Here's how the part is built. I have some questions about the finished solid (model axes, mm). A direction names the side the tool comes from. Give positions to 0.01 mm unless a question says otherwise; leave off trailing zeros. Loops run counter-clockwise (first coordinate to the right, second up) from the corner with the lowest first, then second, coordinate; pieces in that order, holes last. Notation, with made-up numbers: (-37, 68.5) - (0, 68.5) arc R27 ccw to (0, 87.5) - close; hole circle Ø9 at (84.5, 36). An arc over 180 degrees is marked (long way). Use one line per item in the form item = value.
from build123d import *

# Parameters (mm, degrees)
BOSS_EXTRUDE1_DEPTH = 72.4
BOSS_EXTRUDE2_DEPTH = 7.3
BOSS_EXTRUDE3_DEPTH = 4.3
SKETCH4_R           = 25
BOSS_EXTRUDE4_DEPTH = 6.5
SKETCH5_R           = 3.25
CUT_EXTRUDE1_DEPTH  = 3
CUT_EXTRUDE2_DEPTH  = 1
SKETCH7_R           = 1.5
CUT_EXTRUDE3_DEPTH  = 1
SKETCH8_R           = 20
CUT_EXTRUDE4_DEPTH  = 10


with BuildPart() as part:
    # Sketch1 → Boss-Extrude1 (new body)
    with BuildSketch(Plane(origin=(0, 0, 0), x_dir=(1, 0, 0), z_dir=(0, 1, 0))):
        with BuildLine():
            ThreePointArc((69.840771002, 70.864970002), (39.3, 72.2), (8.759228998, 70.864970002))
            ThreePointArc((8.759228998, 70.864970002), (3.821292476, 68.573105669), (1.493169033, 63.652160592))
            ThreePointArc((1.493169033, 63.652160592), (0.466996736, 49.89123235), (0, 36.1))
            ThreePointArc((0, 36.1), (0.466996736, 22.30876765), (1.493169033, 8.547839408))
            ThreePointArc((1.493169033, 8.547839408), (3.821292476, 3.626894331), (8.759228998, 1.335029998))
            ThreePointArc((8.759228998, 1.335029998), (39.3, 0), (69.840771002, 1.335029998))
            ThreePointArc((69.840771002, 1.335029998), (74.778707524, 3.626894331), (77.106830967, 8.547839408))
            ThreePointArc((77.106830967, 8.547839408), (78.133003264, 22.30876765), (78.6, 36.1))
            ThreePointArc((78.6, 36.1), (78.133003264, 49.89123235), (77.106830967, 63.652160592))
            ThreePointArc((77.106830967, 63.652160592), (74.778707524, 68.573105669), (69.840771002, 70.864970002))
        make_face()
    extrude(amount=BOSS_EXTRUDE1_DEPTH)

    # Sketch2 → Boss-Extrude2 (add)
    with BuildSketch(Plane(origin=(0, 72.4, 0), x_dir=(1, 0, 0), z_dir=(0, 1, 0))):
        with BuildLine():
            ThreePointArc((69.66625231, 68.872598745), (39.3, 70.2), (8.93374769, 68.872598745))
            ThreePointArc((8.93374769, 68.872598745), (5.230295298, 67.153700495), (3.484202716, 63.462991687))
            ThreePointArc((3.484202716, 63.462991687), (2.464800099, 49.796540149), (2.000184882, 36.1))
            ThreePointArc((2.000184882, 36.1), (2.464800099, 22.403459851), (3.484202716, 8.737008313))
            ThreePointArc((3.484202716, 8.737008313), (5.230295298, 5.046299505), (8.93374769, 3.327401255))
            ThreePointArc((8.93374769, 3.327401255), (39.3, 2), (69.66625231, 3.327401255))
            ThreePointArc((69.66625231, 3.327401255), (73.369704702, 5.046299505), (75.115797284, 8.737008313))
            ThreePointArc((75.115797284, 8.737008313), (76.135199901, 22.403459851), (76.599815118, 36.1))
            ThreePointArc((76.599815118, 36.1), (76.135199901, 49.796540149), (75.115797284, 63.462991687))
            ThreePointArc((75.115797284, 63.462991687), (73.369704702, 67.153700495), (69.66625231, 68.872598745))
        make_face()
    extrude(amount=BOSS_EXTRUDE2_DEPTH)

    # Sketch3 → Boss-Extrude3 (add)
    with BuildSketch(Plane.XZ):
        with BuildLine():
            ThreePointArc((69.66625231, -3.327401255), (39.3, -2), (8.93374769, -3.327401255))
            ThreePointArc((8.93374769, -3.327401255), (5.230295298, -5.046299505), (3.484202716, -8.737008313))
            ThreePointArc((3.484202716, -8.737008313), (2.464800099, -22.403459851), (2.000184882, -36.1))
            ThreePointArc((2.000184882, -36.1), (2.464800099, -49.796540149), (3.484202716, -63.462991687))
            ThreePointArc((3.484202716, -63.462991687), (5.230295298, -67.153700495), (8.93374769, -68.872598745))
            ThreePointArc((8.93374769, -68.872598745), (39.3, -70.2), (69.66625231, -68.872598745))
            ThreePointArc((69.66625231, -68.872598745), (73.369704702, -67.153700495), (75.115797284, -63.462991687))
            ThreePointArc((75.115797284, -63.462991687), (76.135199901, -49.796540149), (76.599815118, -36.1))
            ThreePointArc((76.599815118, -36.1), (76.135199901, -22.403459851), (75.115797284, -8.737008313))
            ThreePointArc((75.115797284, -8.737008313), (73.369704702, -5.046299505), (69.66625231, -3.327401255))
        make_face()
    extrude(amount=BOSS_EXTRUDE3_DEPTH)

    # Sketch4 → Boss-Extrude4 (add)
    with BuildSketch(Plane.XZ.offset(4.3)):
        with Locations((39.3, -36.1)):
            Circle(SKETCH4_R)
    extrude(amount=BOSS_EXTRUDE4_DEPTH)

    # Sketch5 → Cut-Extrude1 (cut)
    with BuildSketch(Plane(origin=(0, 79.7, 0), x_dir=(1, 0, 0), z_dir=(0, 1, 0))):
        with Locations((69.3, 58.6)):
            Circle(SKETCH5_R)
        with Locations((69.3, 13.6)):
            Circle(SKETCH5_R)
        with Locations((9.3, 13.6)):
            Circle(SKETCH5_R)
        with Locations((9.3, 58.6)):
            Circle(SKETCH5_R)
    extrude(amount=-CUT_EXTRUDE1_DEPTH, mode=Mode.SUBTRACT)

    # Sketch6 → Cut-Extrude2 (cut)
    with BuildSketch(Plane(origin=(0, 79.7, 0), x_dir=(1, 0, 0), z_dir=(0, 1, 0))):
        with BuildLine():
            Line((10.8, 54.1), (67.8, 54.1))
            ThreePointArc((67.8, 54.1), (69.567766953, 53.367766953), (70.3, 51.6))
            Line((70.3, 51.6), (70.3, 20.6))
            ThreePointArc((70.3, 20.6), (69.567766953, 18.832233047), (67.8, 18.1))
            Line((67.8, 18.1), (10.8, 18.1))
            ThreePointArc((10.8, 18.1), (9.032233047, 18.832233047), (8.3, 20.6))
            Line((8.3, 20.6), (8.3, 51.6))
            ThreePointArc((8.3, 51.6), (9.032233047, 53.367766953), (10.8, 54.1))
        make_face()
    extrude(amount=-CUT_EXTRUDE2_DEPTH, mode=Mode.SUBTRACT)

    # Sketch7 → Cut-Extrude3 (cut)
    with BuildSketch(Plane(origin=(0, 79.7, 0), x_dir=(1, 0, 0), z_dir=(0, 1, 0))):
        with Locations((32.8, 12.1)):
            Circle(SKETCH7_R)
        with Locations((45.8, 12.1)):
            Circle(SKETCH7_R)
    extrude(amount=-CUT_EXTRUDE3_DEPTH, mode=Mode.SUBTRACT)

    # Sketch8 → Cut-Extrude4 (cut)
    with BuildSketch(Plane.XZ.offset(10.8)):
        with Locations((39.3, -36.1)):
            Circle(SKETCH8_R)
    extrude(amount=-CUT_EXTRUDE4_DEPTH, mode=Mode.SUBTRACT)


solid = part.part
(1) For P1, Ø2.5, axis at x = 32.8, z = -12.1, coming from the +Y side; P2, Ø0.8, axis at x = 48.5, y = 79, coming from the -Z side; P3, Ø12, axis at x = 40.5, z = -35.5, coming from the -Y side, each with a flat end and sliding along its axis, tell me the tip position at first contact or that it passes through.
Geometry says:
P1 = 78.7
P2 = -70.09
P3 = -0.8
(2) If we section it at A-A (x = 39.3): List the corners of the cut face in (y, z) for me.
Geometry says:
outline = (-10.8, -61.1) - (-4.3, -61.1) - (-4.3, -70.2) - (0, -70.2) - (0, -72.2) - (72.4, -72.2) - (72.4, -70.2) - (79.7, -70.2) - (79.7, -54.1) - (78.7, -54.1) - (78.7, -18.1) - (79.7, -18.1) - (79.7, -2) - (72.4, -2) - (72.4, 0) - (0, 0) - (0, -2) - (-4.3, -2) - (-4.3, -11.1) - (-10.8, -11.1) - (-10.8, -16.1) - (-0.8, -16.1) - (-0.8, -56.1) - (-10.8, -56.1) - close
(3) For faces 5 (the cylindrical face through (36.045, -7.504, -11.313)), 6 (the cylindrical face through (72.4, 78.22, -14.58)), 7 (the cylindrical face through (2.475, 75.999, -49.988)), 8 (the cylindrical face through (2.454, -2.12, -49.605)), which set-ups out of +Z, -Z, +X, -X, +Y, -Y let a thin tool reach every point of the face, with its end or its side?
Geometry says:
face_5 = -Y
face_6 = +Y
face_7 = -Z, -X, +Y
face_8 = -Z, -X, -Y
(4) If we section it at B-B (z = -5): List the corners of the cut face in (x, y) for me.
Geometry says:
outline = (2.71, 0) - (5.28, 0) - (5.28, -4.3) - (73.32, -4.3) - (73.32, 0) - (75.89, 0) - (75.89, 72.4) - (73.32, 72.4) - (73.32, 79.7) - (5.28, 79.7) - (5.28, 72.4) - (2.71, 72.4) - close
(5) Thinking about a two-plate mould opening in Z: for faces 1 (the cylindrical face through (47, 79, -13)), 2 (the cylindrical face through (76.125, 75.999, -22.212)), 3 (the flat face through (39, -0.8, -36)), 4 (the cylindrical face through (73.411, 75.999, -67.112)), which applies, pulls with the +Z half, pulls with the -Z half, needs draft (parallel to the pull), parting line crosses it, or undercut?
Geometry says:
face_1 = undercut
face_2 = pulls with the +Z half
face_3 = undercut
face_4 = pulls with the -Z half
(6) If we section it at D-D (z = -34): List the corners of the cut face in (x, y) for me.
Geometry says:
outline = (0.03, 0) - (2.04, 0) - (2.04, -4.3) - (14.39, -4.3) - (14.39, -10.8) - (19.41, -10.8) - (19.41, -0.8) - (59.19, -0.8) - (59.19, -10.8) - (64.21, -10.8) - (64.21, -4.3) - (76.56, -4.3) - (76.56, 0) - (78.57, 0) - (78.57, 72.4) - (76.56, 72.4) - (76.56, 79.7) - (70.3, 79.7) - (70.3, 78.7) - (8.3, 78.7) - (8.3, 79.7) - (2.04, 79.7) - (2.04, 72.4) - (0.03, 72.4) - close
(7) If I drill on probe 1 along Z at (x, y) = (32, 79); probe 2 along X at (y, z) = (77, -13); probe 3 along Z at (x, y) = (9.3, 77.4), over which ranges is the centre line in solid material (lowest first)?
Geometry says:
probe_1 = -70.12 to -54.1, -18.1 to -13.37, -10.83 to -2.08
probe_2 = 3.11 to 6.11, 12.49 to 66.11, 72.49 to 75.49
probe_3 = -68.9 to -61.85, -55.35 to -16.85, -10.35 to -3.3
(8) If we section it at C-C (y = 16): List the corners of the cut face in (x, z) for me.
Geometry says:
outline = (0, -36.1) arc R340.03 ccw to (1.49, -63.65) arc R8 ccw to (8.76, -70.86) arc R350 ccw to (69.84, -70.86) arc R8 ccw to (77.11, -63.65) arc R340.03 ccw to (78.6, -36.1) arc R340.03 ccw to (77.11, -8.55) arc R8 ccw to (69.84, -1.34) arc R350 ccw to (8.76, -1.34) arc R8 ccw to (1.49, -8.55) arc R340.03 ccw to start
